Geometry: final body of the model. Coordinates: model frame, mm. Face numbers are marked on the shaded views. Coordinates: 2 decimals unless noted, no trailing zeros. Order: outer loops, then holes, each group sorted by start corner. A loop starts at its lowest first (then second) coordinate and runs counter-clockwise, first axis right, second up. Notation, with made-up numbers: (39, 83) - (96, 83) arc R18 ccw to (96, 103) - close; hole circle Ø10 at (78, 54). An arc over 180 degrees is marked (long way). Use a Markdown table: item, result. Add a question column.
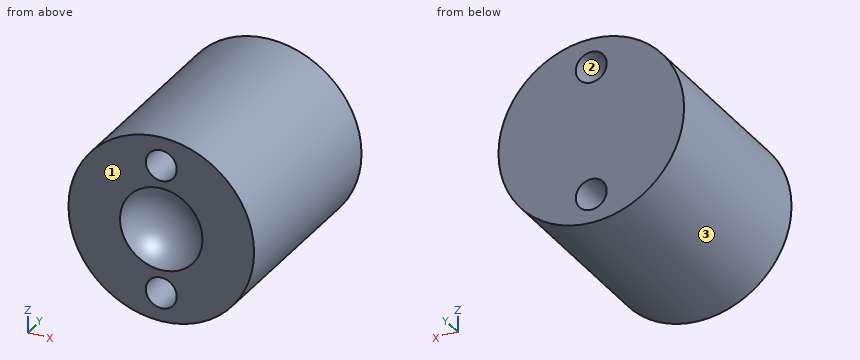
Autodesk Inventor part; units mm, degrees
ref_plane "YZ Plane" through (0, 0, 0) normal (1, 0, 0) x (0, 1, 0)
ref_plane "XZ Plane" through (0, 0, 0) normal (0, 1, 0) x (-1, 0, 0)
ref_plane "XY Plane" through (0, 0, 0) normal (0, 0, 1) x (1, 0, 0)
sketch "Boceto1" plane through (0, 0, 0) normal (0, 1, 0) x (-1, 0, 0)
  circle A0 centre (0, 0) radius 9
  dimension "d0" = 18
extrude "Extrusión1" add sketch "Boceto1" against normal blind 20
sketch "Boceto3" plane through (0, 0, 0) normal (0, 1, 0) x (1, 0, 0)
  point P0 (0, 0)
sketch "Boceto4" plane through (0, 0, 0) normal (0, 1, 0) x (1, 0, 0)
  circle A0 centre (0, -6.226) radius 1.5
  circle A1 centre (0, 6.226) radius 1.5
  point P0 (0, 0)
  dimension "d6" = 3
  dimension "d7" = 3
extrude "Extrusión2" cut sketch "Boceto4" against normal blind 20
sketch "Boceto5" plane through (0, -20, 0) normal (0, -1, 0) x (1, 0, 0)
  arc A0 (0, 4) -> (0, -4) centre (0, 0) ccw
  line L0 (0, 4) -> (0, -4)
  dimension "d12" = 8
revolve "Revolución3" cut sketch "Boceto5" angle 360 about axis through (0, -20, 4) along (0, 0, -1)
properties part number "rueda loca"
1) Section query D-D (x = -3). Return the cut outline in (y, z), and give its area (3 significant figures).
2) First-contact query: pin 1 (3 mm diameter, centred on y = -10.5, z = 6.5, fed in from +X); pin 2 (1 mm diameter, centred on x = 0.5, y = -8.5, fed in from +Z); pin 3 (1 mm diameter, centred on y = -6, z = 2.5, fed in from -X); pin 4 (6 mm diameter, centred on x = -5.5, y = -6, fed in from +Z). Flat tips, straight axial feed; report the tip coordinate or a pass-through.
3) Line query: line 1 (Z direction, x = 0, y = -8.75); line 2 (X direction, y = -1, z = -7.5); line 3 (X direction, y = -14, z = 7). Output: solid intervals per line, ascending. Write a range as from..to.
4) Section query C-C (z = 0). Return the cut outline in (x, y), and give its area (3 significant figures).
5) Section query B-B (z = 7.25). Return the cut outline in (x, y).
6) Section query A-A (x = 0). Return the cut outline in (y, z).
7) Draft query along Z for the marked faces 1, 2 and 3. Return one class per face: released by +Z, released by -Z, zero draft, split by the parting line, or undercut.
From the geometry:
| question | item | result |
|---|---|---|
| 1 | outline | (-20, -8.49) - (0, -8.49) - (0, 8.49) - (-20, 8.49) - (-20, 2.65) arc R2.65 cw to (-20, -2.65) - close |
| 1 | area | 328 mm^2 |
| 2 | pin 1 | stops at x = 7.48 |
| 2 | pin 2 | stops at z = 9 |
| 2 | pin 3 | stops at x = -8.77 |
| 2 | pin 4 | stops at z = 8.65 |
| 3 | line 1 | z = -9..-7.73, -4.73..4.73, 7.73..9 |
| 3 | line 2 | x = -4.97..-0.79, 0.79..4.97 |
| 3 | line 3 | x = -5.66..-1.28, 1.28..5.66 |
| 4 | outline | (-9, -20) - (-4, -20) arc R4 cw to (4, -20) - (9, -20) - (9, 0) - (-9, 0) - close |
| 4 | area | 335 mm^2 |
| 5 | outline | (-5.33, -20) - (-1.1, -20) - (-1.1, 0) - (-5.33, 0) - close; (1.1, -20) - (5.33, -20) - (5.33, 0) - (1.1, 0) - close |
| 6 | outline | (-20, -9) - (0, -9) - (0, -7.73) - (-20, -7.73) - close; (-20, -4.73) - (0, -4.73) - (0, 4.73) - (-20, 4.73) - (-20, 4) arc R4 cw to (-20, -4) - close; (-20, 7.73) - (0, 7.73) - (0, 9) - (-20, 9) - close |
| 7 | face 1 | zero draft |
| 7 | face 2 | undercut |
| 7 | face 3 | split by the parting line |
